```python
from build123d import *

# Parameters (mm, degrees)
SKETCH1_W                                           = 41
SKETCH1_H                                           = 25
BOSS_EXTRUDE1_DEPTH                                 = 13
SKETCH2_R                                           = 1.5
CUT_EXTRUDE1_DEPTH                                  = 50.749371855
LPATTERN1_COUNT                                     = 2
LPATTERN1_PITCH                                     = 10
LPATTERN3_COUNT                                     = 2
LPATTERN3_PITCH                                     = 21
SKETCH8_R                                           = 1.5
CUT_EXTRUDE5_DEPTH                                  = 8
SKETCH3_R                                           = 7.525
CUT_EXTRUDE2_DEPTH                                  = 6.1
CBORE_FOR_M3_HEX_SOCKET_HEAD_CAP_SCREW1_D           = 3.4
CBORE_FOR_M3_HEX_SOCKET_HEAD_CAP_SCREW1_CBORE_D     = 6
CBORE_FOR_M3_HEX_SOCKET_HEAD_CAP_SCREW1_CBORE_DEPTH = 3.4
FILLET1_R                                           = 20
CUT_EXTRUDE4_DEPTH                                  = 50.749371855
CUT_EXTRUDE4_DEPTH_BACK                             = 50.749371855
BOSS_EXTRUDE3_START                                 = 0.2
BOSS_EXTRUDE3_DEPTH                                 = 0.2
LPATTERN2_COUNT                                     = 2
LPATTERN2_PITCH                                     = 24.09


with BuildPart() as part:
    # Sketch1 → Boss-Extrude1 (new body)
    with BuildSketch(Plane(origin=(0, 0, 0), x_dir=(1, 0, 0), z_dir=(0, 1, 0))):
        with Locations((20.5, 12.5)):
            Rectangle(SKETCH1_W, SKETCH1_H)
    extrude(amount=BOSS_EXTRUDE1_DEPTH)

    # Sketch2 → Cut-Extrude1 (cut, through all)
    with BuildSketch(Plane.XY):
        with Locations((5, 4.545)):
            Circle(SKETCH2_R)
    cut_extrude1 = extrude(amount=-CUT_EXTRUDE1_DEPTH, mode=Mode.SUBTRACT)

    # LPattern1: Cut-Extrude1 ×2
    with Locations(*[(i * LPATTERN1_PITCH, 0, 0) for i in range(1, LPATTERN1_COUNT)]):
        add(cut_extrude1, mode=Mode.SUBTRACT)

    # LPattern3: Cut-Extrude1 ×2
    with Locations(*[(i * LPATTERN3_PITCH, 0, 0) for i in range(1, LPATTERN3_COUNT)]):
        add(cut_extrude1, mode=Mode.SUBTRACT)

    # Sketch8 → Cut-Extrude5 (cut)
    with BuildSketch(Plane.XY):
        with Locations((36, 4.545)):
            Circle(SKETCH8_R)
    extrude(amount=-CUT_EXTRUDE5_DEPTH, mode=Mode.SUBTRACT)

    # Sketch3 → Cut-Extrude2 (cut)
    with BuildSketch(Plane(origin=(0, 13, 0), x_dir=(1, 0, 0), z_dir=(0, 1, 0))):
        with Locations((10.16, 12.135)):
            Circle(SKETCH3_R)
        with BuildLine():
            Line((34.25, 8.335), (10.16, 8.335))
            ThreePointArc((10.16, 8.335), (6.36, 12.135), (10.16, 15.935))
            Line((10.16, 15.935), (34.25, 15.935))
            ThreePointArc((34.25, 15.935), (38.05, 12.135), (34.25, 8.335))
        make_face()
        with BuildLine():
            Line((10.16, 4.61), (6.635, 4.61))
            ThreePointArc((6.635, 4.61), (3.806572875, 5.781572875), (2.635, 8.61))
            Line((2.635, 8.61), (2.635, 15.66))
            ThreePointArc((2.635, 15.66), (3.806572875, 18.488427125), (6.635, 19.66))
            Line((6.635, 19.66), (10.16, 19.66))
            Line((10.16, 19.66), (10.16, 4.61))
        make_face()
    extrude(amount=-CUT_EXTRUDE2_DEPTH, mode=Mode.SUBTRACT)

    # CBORE for M3 Hex Socket Head Cap Screw1 (through all)
    with Locations(Plane(origin=(0, 0, 0), x_dir=(-1, 0, 0), z_dir=(0, -1, 0))):
        with Locations((-34.25, 12.135), (-10.16, 12.135)):
            CounterBoreHole(CBORE_FOR_M3_HEX_SOCKET_HEAD_CAP_SCREW1_D / 2, CBORE_FOR_M3_HEX_SOCKET_HEAD_CAP_SCREW1_CBORE_D / 2, CBORE_FOR_M3_HEX_SOCKET_HEAD_CAP_SCREW1_CBORE_DEPTH)

    # Fillet1
    fillet1_edges = [part.edges().sort_by_distance(p)[0] for p in [
        (16.655046189, 9.95, -15.935),
        (16.655046189, 9.95, -8.335),
    ]]
    fillet(fillet1_edges, radius=FILLET1_R)

    # Sketch7 → Cut-Extrude4 (cut, two sides: drawn at the far end of the back side and taken through both)
    with BuildSketch(Plane.ZY.offset(-CUT_EXTRUDE4_DEPTH_BACK)):
        Polygon((-50.521542775, 74.251702659), (-25, 13), (-20, 1), (-20, 0), (-20, -66.356011214), (-149.691728644, -94.508034559), (-180.213271419, 46.099679315), align=None)
    extrude(amount=CUT_EXTRUDE4_DEPTH + CUT_EXTRUDE4_DEPTH_BACK, mode=Mode.SUBTRACT)

    # Sketch9 → Boss-Extrude3 (add)
    with BuildSketch(Plane.XZ.offset(-3.4).offset(BOSS_EXTRUDE3_START)):
        with BuildLine():
            Line((8.46, -14.606841419), (8.46, -9.663158581))
            ThreePointArc((8.46, -9.663158581), (7.16, -12.135), (8.46, -14.606841419))
        make_face()
        with BuildLine():
            ThreePointArc((13.16, -12.135), (12.815183609, -10.738575996), (11.86, -9.663158581))
            Line((11.86, -9.663158581), (11.86, -14.606841419))
            ThreePointArc((11.86, -14.606841419), (12.815183609, -13.531424004), (13.16, -12.135))
        make_face()
    boss_extrude3 = extrude(amount=-BOSS_EXTRUDE3_DEPTH)

    # LPattern2: Boss-Extrude3 ×2
    with Locations(*[(i * LPATTERN2_PITCH, 0, 0) for i in range(1, LPATTERN2_COUNT)]):
        add(boss_extrude3)


solid = part.part
```
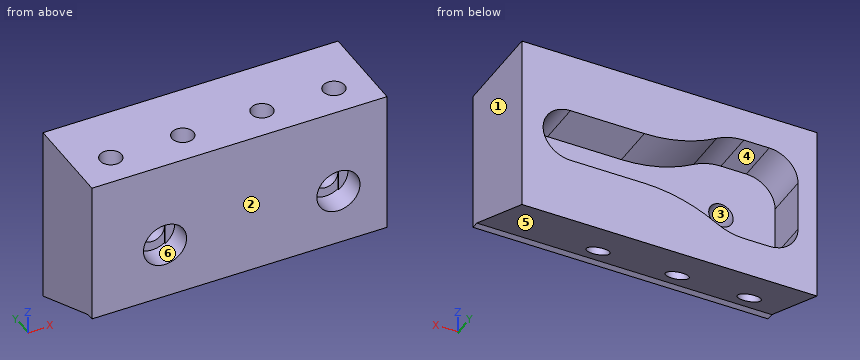
CAD build for the part. Positions are in the model's coordinates, mm. Face numbers are marked on the shaded views. A direction names the side the tool comes from. Give positions to 0.01 mm unless a question says otherwise; leave off trailing zeros. Write each loop counter-clockwise with the first axis right and the second up, starting at its lowest first coordinate (ties: lowest second). Pieces come first, ordered by that corner, then holes. Notation, with made-up numbers: M -27,44 L 23,44 A26 cw 23,74 Z; hole C -40,64 d6. An arc over 180 degrees is marked long. Return JSON: item names as keys, results as strings. Group by question number.
(1) Band-saw the part on B-B (y = 2). Give the cut face in (x, z) (3 decimals).
(2) Band-saw the part on A-A (x = 5). Give the cut face in (y, z) (3 decimals), and give its area (3 significant figures).
(3) Mould opens along X. For the marked faces 1, 2 and 3 say: pulls with the +X half, pulls with the -X half, needs draft (parallel to the pull), parting line crosses it, or undercut.
(4) Flat gauge pins, fed straight in: pin 1 Ø1 at (x, y) = (30, 11) entering from -Z (3 decimals); pin 2 Ø2.5 at (x, y) = (5, 4.545) entering from +Z; pin 3 Ø4 at (x, y) = (17.5, 5.5) entering from -Z; pin 4 Ø0.8 at (x, y) = (13.5, 0.5) entering from -Z. Where does each tip first touch, or does it go through?
(5) 3-axis set-ups, long thin cutter, end or side, ignore diameter. For the marked faces 4, 5 and 6: which of +Z, -Z, +X, -X, +Y, -Y reach the whole face in a straight line?
(6) Drill centre lines: L1, parallel to X at y = 4.5, z = -17.5; L2, parallel to Y at x = 36, z = -1.75 (3 decimals); L3, parallel to X at y = 3, z = -9.5. Where is each one in solid material? Low to high. Write a range as [from, to].
(7) Band-saw the part on C-C (z = -6.75). Give the cut face in (x, y) (3 decimals).
Entries:
{
 "1": {"outline": "M 0,-20.417 L 41,-20.417 L 41,0 L 0,0 Z; hole C 10.16,-12.135 d6; hole C 34.25,-12.135 d6"},
 "2": {"outline": "M 0,-20 L 1,-20 L 3.045,-20.852 L 3.045,0 L 0,0 Z; M 6.045,-22.102 L 13,-25 L 13,-19.311 L 6.9,-19.311 L 6.9,-4.959 L 13,-4.959 L 13,0 L 6.045,0 Z", "area": "138 mm^2"},
 "3": {"face 1": "pulls with the +X half", "face 2": "needs draft", "face 3": "undercut"},
 "4": {"pin 1": "stops at z = -24.375", "pin 2": "passes through", "pin 3": "stops at z = -22.71", "pin 4": "stops at z = -20"},
 "5": {"face 4": "+Y", "face 5": "-Z, +X, -X, -Y", "face 6": "-Y"},
 "6": {"L1": "x = [0, 3.5], [6.5, 13.5], [16.5, 24.5], [27.5, 41]", "L2": "y = [0, 3.045], [6.045, 13]", "L3": "x = [0, 8.73], [11.59, 32.82], [35.68, 41]"},
 "7": {"outline": "M 0,0 L 41,0 L 41,13 L 16.184,13 L 16.184,6.9 L 3.094,6.9 L 3.094,13 L 0,13 Z; hole C 5,4.545 d3; hole C 15,4.545 d3; hole C 26,4.545 d3; hole C 36,4.545 d3"}
}
